Design review of the part built by this model. Coordinates are the model's own, in mm. Face numbers are marked on the shaded views. A direction names the side the tool comes from. Coordinates: 2 decimals unless noted, no trailing zeros. Write each loop counter-clockwise with the first axis right and the second up, starting at its lowest first coordinate (ties: lowest second). Pieces come first, ordered by that corner, then holes. Notation, with made-up numbers: (-8.5, 7) -> (4.5, 7) arc R13 cw to (4.5, 17) -> close; hole circle Ø3 at (83.25, 88). An arc over 180 degrees is marked (long way). Write item = value, one per line. Start each with the question number.
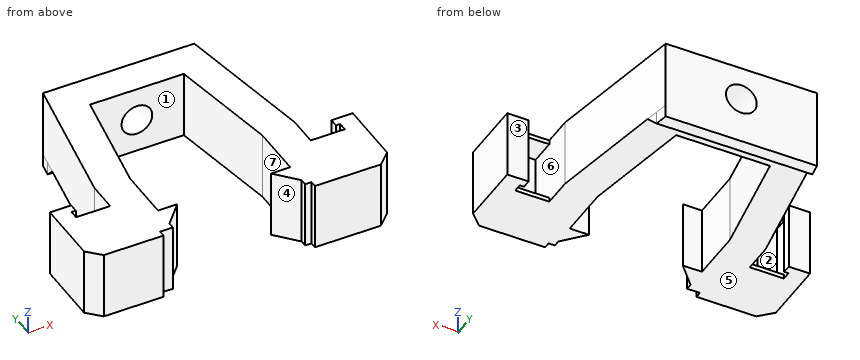
```python
from build123d import *

# Parameters (mm, degrees)
BOSS_EXTRUDE1_DEPTH = 8
SKETCH2_R           = 1.8
CUT_EXTRUDE1_DEPTH  = 31.60183818
BOSS_EXTRUDE4_DEPTH = 8
BOSS_EXTRUDE5_DEPTH = 0.5
BOSS_EXTRUDE6_START = -8
BOSS_EXTRUDE6_DEPTH = 0.5
BOSS_EXTRUDE3_DEPTH = 1.5
CHAMFER3_SIZE       = 1.5


with BuildPart() as part:
    # Sketch1 → Boss-Extrude1 (new body)
    with BuildSketch(Plane.XY):
        Polygon((8.867161478, 0), (-8.867161478, 0), (-11.75, -16.656400352), (-11.75, -27.1), (-9.25, -27.1), (-9.25, -26.35), (-7.75, -26.35), (-7.75, -25.6), (-5.5, -23.1), (-7.75, -23.1), (-7.75, -17), (-5.5, -4), (5.5, -4), (7.75, -17), (7.75, -23.1), (5.5, -23.1), (7.75, -25.6), (7.75, -26.35), (8.5, -26.35), (8.5, -27.1), (11.75, -27.1), (11.75, -16.656400352), align=None)
    extrude(amount=BOSS_EXTRUDE1_DEPTH)

    # Sketch2 → Cut-Extrude1 (cut, through all)
    with BuildSketch(Plane(origin=(0, 0, 0), x_dir=(1, 0, 0), z_dir=(0, 1, 0))):
        with Locations(Location((0, -4, 0), (0, 0, 180))):
            Circle(SKETCH2_R)
    extrude(amount=-CUT_EXTRUDE1_DEPTH, mode=Mode.SUBTRACT)

    # Sketch7 → Boss-Extrude4 (add)
    with BuildSketch(Plane(origin=(0, 0, 0), x_dir=(-1, 0, 0), z_dir=(0, 0, -1))):
        Polygon((-11.75, -27.1), (-16.25, -27.1), (-17.75, -25.6), (-17.75, -18.1), (-15.25, -18.1), (-15.25, -19.1), (-15.75, -19.1), (-15.75, -21.6), (-14.25, -23.1), (-11.75, -23.1), align=None)
        Polygon((16.25, -27.1), (17.75, -25.6), (17.75, -18.1), (15.25, -18.1), (15.25, -19.1), (15.75, -19.1), (15.75, -21.6), (14.25, -23.1), (11.75, -23.1), (11.75, -27.1), align=None)
    extrude(amount=-BOSS_EXTRUDE4_DEPTH)

    # Sketch8 → Boss-Extrude5 (add)
    with BuildSketch(Plane(origin=(0, 0, 0), x_dir=(-1, 0, 0), z_dir=(0, 0, -1))):
        Polygon((-11.75, -23.1), (-11.75, -20.1), (-15.75, -20.1), (-15.75, -21.6), (-14.25, -23.1), align=None)
        Polygon((15.75, -20.1), (11.75, -20.1), (11.75, -23.1), (14.25, -23.1), (15.75, -21.6), align=None)
    extrude(amount=-BOSS_EXTRUDE5_DEPTH)

    # Sketch8<2> → Boss-Extrude6 (add)
    with BuildSketch(Plane(origin=(0, 0, 0), x_dir=(-1, 0, 0), z_dir=(0, 0, -1)).offset(BOSS_EXTRUDE6_START)):
        Polygon((-11.75, -23.1), (-11.75, -20.1), (-15.75, -20.1), (-15.75, -21.6), (-14.25, -23.1), align=None)
        Polygon((15.75, -20.1), (11.75, -20.1), (11.75, -23.1), (14.25, -23.1), (15.75, -21.6), align=None)
    extrude(amount=BOSS_EXTRUDE6_DEPTH)

    # Sketch5 → Boss-Extrude3 (add)
    with BuildSketch(Plane(origin=(0, 0, 0), x_dir=(-1, 0, 0), z_dir=(0, 0, -1))):
        Polygon((8.867161478, 0), (-8.867161478, 0), (-9.126776862, -1.5), (9.126776862, -1.5), align=None)
    extrude(amount=BOSS_EXTRUDE3_DEPTH)

    # Chamfer3
    # the kernel refuses this chamfer: 1.5 mm, written as the material it adds along each edge
    with BuildSketch(Plane(origin=(12.984301344, -1.5, 0), x_dir=(0, -0.9996219169112969, 0.02749587661058638), z_dir=(-1, 0, 0))) as chamfer3_piece_1_section:
        Polygon((CHAMFER3_SIZE * 0.999621916911, -CHAMFER3_SIZE * 0.0274958766106), (-CHAMFER3_SIZE * 0.0274958766106, -CHAMFER3_SIZE * 0.999621916911), (0, 0), align=None)
    chamfer3_piece_1 = extrude(amount=25.968602688, mode=Mode.PRIVATE)
    chamfer3_piece_1 = split(chamfer3_piece_1, bisect_by=Plane(origin=(-8.945746351, -0.454045937, -0.498825905), z_dir=(0.9853505058554479, -0.17054143370575114, 0)), keep=Keep.TOP, mode=Mode.PRIVATE)
    chamfer3_piece_1 = split(chamfer3_piece_1, bisect_by=Plane(origin=(8.945746351, -0.454045937, -0.498825905), z_dir=(-0.9853505058554478, -0.17054143370575137, 0)), keep=Keep.TOP, mode=Mode.PRIVATE)
    add(chamfer3_piece_1)
    # the kernel refuses this chamfer: 1.5 mm, written as the material it takes off along each edge


solid = part.part
```
(1) Mouldability with a two-part tool opening along Y and no side actions: class the marked faces 1, 2 and 3 as pulls with the +Y half, pulls with the -Y half, needs draft (parallel to the pull), parting line crosses it, or undercut.
(2) For line 1 (Z direction, x = 0, y = -0.95); line 2 (X direction, y = -23.5, z = 5.25); line 3 (Z direction, x = 0, y = -1.9), list the stretches that pass through material, from the lowest coordinate up.
(3) For the marked faces 4, 5, 6 and 7, list the 3-axis set-ups (+Z, -Z, +X, -X, +Y, -Y) from which the entire face can be reached by the end or side of a thin tool; tool diameter is ignored.
(4) Take a section at C-C, the plane x = -5. State the section outline as (y, z) points.
(5) For pin 1 Ø2 at (x, y) = (11.5, -20.5) entering from -Z; pin 2 Ø3 at (x, z) = (-13.5, 5) entering from +Y; pin 3 Ø0.6 at (y, z) = (-26.5, 3.5) entering from -X, all flat-tipped, find the tip position at first contact; note any pin that passes through.
(6) Take a section at A-A, the plane x = 0. State the section outline as (y, z) points, then the cut area to 3 significant figures.
(7) Take a section at B-B, the plane x = -13. State the section outline as (y, z) points, then the cut area to 3 significant figures.
(8) Take a section at D-D, the plane x = 10. State the section outline as (y, z) points.
Report:
q1.face_1 = pulls with the -Y half
q1.face_2 = undercut
q1.face_3 = pulls with the +Y half
q2.line_1 = -1.5 to 2.2, 5.8 to 8
q2.line_2 = -17.75 to -5.86, 5.86 to 17.75
q2.line_3 = -1.1 to 2.2, 5.8 to 8
q3.face_4 = +Z, -Z, -Y
q3.face_5 = -Z, +X, -X, -Y
q3.face_6 = +Y
q3.face_7 = +Z, -Z
q4.outline = (-4, 0) -> (-3, 0) -> (-1.5, -1.5) -> (0, -1.5) -> (0, 8) -> (-4, 8) -> close
q5.pin_1 = 0
q5.pin_2 = -22.35
q5.pin_3 = -17.15
q6.outline = (-4, 0) -> (-3, 0) -> (-1.5, -1.5) -> (0, -1.5) -> (0, 2.2) -> (-4, 2.2) -> close; (-4, 5.8) -> (0, 5.8) -> (0, 8) -> (-4, 8) -> close
q6.area = 21.0 mm2
q7.outline = (-27.1, 0) -> (-20.1, 0) -> (-20.1, 0.5) -> (-23.1, 0.5) -> (-23.1, 7.5) -> (-20.1, 7.5) -> (-20.1, 8) -> (-27.1, 8) -> close
q7.area = 35.0 mm2
q8.outline = (-27.1, 0) -> (-6.55, 0) -> (-6.55, 8) -> (-27.1, 8) -> close
